```python
from build123d import *

# Parameters (mm, degrees)
BOX012_W                  = 5
BOX012_H                  = 5
BOX012_DEPTH              = 6.66667
ARRAY_X_COUNT             = 2
ARRAY_X_PITCH             = 45
ARRAY_Y_COUNT             = 2
ARRAY_Y_PITCH             = 65
BOX011_W                  = 50
BOX011_H                  = 70
BOX011_DEPTH              = 10
FUSION003_PLACEMENT_ANGLE = 90


with BuildPart() as obj1:
    # Box012 → Box012 (new body)
    with BuildSketch(Plane(origin=(30, 20, 0), x_dir=(1, 0, 0), z_dir=(0, 0, 1))):
        with Locations((2.5, 2.5)):
            Rectangle(BOX012_W, BOX012_H)
    extrude(amount=BOX012_DEPTH)

    # Array X: obj1_2


with BuildPart() as obj1_1:
    add(obj1.part)
    with Locations(*[(i * ARRAY_X_PITCH, 0, 0) for i in range(1, ARRAY_X_COUNT)]):
        add(obj1.part)

    # Array Y: obj1_2


with BuildPart() as obj1_2:
    add(obj1_1.part)
    with Locations(*[(0, i * ARRAY_Y_PITCH, 0) for i in range(1, ARRAY_Y_COUNT)]):
        add(obj1_1.part)


with BuildPart() as fusion003:
    # Box011 → Box011 (new body)
    with BuildSketch(Plane(origin=(30, 20, 6.66667), x_dir=(1, 0, 0), z_dir=(0, 0, 1))):
        with Locations((25, 35)):
            Rectangle(BOX011_W, BOX011_H)
    extrude(amount=BOX011_DEPTH)

    # Fusion003: union obj1
    add(obj1_2.part)


with BuildPart() as fusion003_1:
    # Fusion003 placement: moved
    add(fusion003.part.moved(Location((210, 0, 97))).rotate(Axis((210, 0, 97), (0, 0, 1)), FUSION003_PLACEMENT_ANGLE))


solid = fusion003_1.part
```
CAD build for the part. Positions are in the model's coordinates, mm. A direction names the side the tool comes from. Round coordinates to 2 decimals unless told otherwise and drop trailing zeros. Order: outer loops, then holes, each group sorted by start corner. A loop starts at its lowest first (then second) coordinate and runs counter-clockwise, first axis right, second up. Notation, with made-up numbers: (-3.75, 70) - (22.25, 70) arc R26 cw to (22.25, 104) - close; hole circle Ø11 at (84.25, 58.25). An arc over 180 degrees is marked (long way). Answer in a Markdown table with one row per item. Add a question column.
(1) Drop a flat-ended pin along its axis: pin 1 Ø4 at (x, y) = (167.5, 39) entering from -Z. Give the stop position or say it passes through.
(2) 3-axis set-ups, long thin cutter, end or side, ignore diameter. For faces 1 (the face through (125, 32, 100)), 2 (the face through (122, 32, 97)), 3 (the face through (188, 35, 100)): which of +Z, -Z, +X, -X, +Y, -Y reach the whole face in a straight line?
(3) Band-saw the part on C-C on x = 163. List the corners of the cut face in (y, z), and give its area (3 significant figures).
(4) Band-saw the part on A-A on z = 99.25. List the corners of the cut face in (x, y), and give its area (3 significant figures).
(5) Probe L1, parallel to Z at x = 155, y = 74.5. List the from-to ranges inside material, lowest first. Write a range as [from, to].
(6) Band-saw the part on B-B on y = 66. List the corners of the cut face in (x, z), and give its area (3 significant figures).
(7) Mould opens along X. For faces 4 (the face through (123, 75, 100)), 5 (the face through (185, 32, 100)), 6 (the face through (185, 77, 100)), 7 (the face through (120, 55, 107)) say: +X half, -X half, draft (parallel to the pull), parting line (faces both ways), or undercut.
Data:
| question | item | result |
|---|---|---|
| 1 | pin 1 | stops at z = 103.67 |
| 2 | face 1 | -Z, +Y, -Y |
| 2 | face 2 | -Z, +X, -X, +Y, -Y |
| 2 | face 3 | -Z, +X, -X |
| 3 | outline | (30, 103.67) - (80, 103.67) - (80, 113.67) - (30, 113.67) - close |
| 3 | area | 500 mm^2 |
| 4 | outline | (120, 30) - (125, 30) - (125, 35) - (120, 35) - close; (120, 75) - (125, 75) - (125, 80) - (120, 80) - close; (185, 30) - (190, 30) - (190, 35) - (185, 35) - close; (185, 75) - (190, 75) - (190, 80) - (185, 80) - close |
| 4 | area | 100 mm^2 |
| 5 | L1 | z = [103.67, 113.67] |
| 6 | outline | (120, 103.67) - (190, 103.67) - (190, 113.67) - (120, 113.67) - close |
| 6 | area | 700 mm^2 |
| 7 | face 4 | draft |
| 7 | face 5 | undercut |
| 7 | face 6 | undercut |
| 7 | face 7 | -X half |
